```python
from build123d import *

# Parameters (mm, degrees)
F0_W     = 63.5
F0_H     = 139.7
F1_DEPTH = 5.207
F2_W     = 5.207
F2_H     = 16.9333164
F2_H_2   = 12.7
F2_H_3   = 19.05
F2_W_2   = 15.875
F2_H_4   = 5.207
F2_W_3   = 12.7
F2_W_4   = 9.525
F3_DEPTH = 5.208


# Not quite as in the source:
# - a feature names something its author has since deleted; it is built from what else it names


with BuildPart() as f1:
    # F0 (on Right) → F1 (new body)
    with BuildSketch(Plane.YZ):
        Rectangle(F0_W, F0_H)
    extrude(amount=F1_DEPTH)

    # F2 (on face) → F3 (cut, through all)
    with BuildSketch(Plane.YZ.offset(5.207)):
        with Locations((-29.1465, 41.3046418)):
            Rectangle(F2_W, F2_H)
        with Locations((-29.1465, 13.7879836)):
            Rectangle(F2_W, F2_H_2)
        with Locations((-29.1465, -11.6120164)):
            Rectangle(F2_W, F2_H_2)
        with Locations((-29.1465, -40.1870164)):
            Rectangle(F2_W, F2_H_3)
        with Locations((-23.8125, -67.2465)):
            Rectangle(F2_W_2, F2_H_4)
        with Locations((3.175, -67.2465)):
            Rectangle(F2_W_3, F2_H_4)
        with Locations((26.9875, -67.2465)):
            Rectangle(F2_W_4, F2_H_4)
        with Locations((26.9875, 67.2465)):
            Rectangle(F2_W_4, F2_H_4)
        with Locations((3.175, 67.2465)):
            Rectangle(F2_W_3, F2_H_4)
        with Locations((-23.8125, 67.2465)):
            Rectangle(F2_W_2, F2_H_4)
    extrude(amount=-F3_DEPTH, mode=Mode.SUBTRACT)


solid = f1.part
```
Could you check a few things on this model? Use its own coordinates, in mm. A direction names the side the tool comes from. Round coordinates to 2 decimals unless told otherwise and drop trailing zeros. Write each loop counter-clockwise with the first axis right and the second up, starting at its lowest first coordinate (ties: lowest second). Pieces come first, ordered by that corner, then holes. Notation, with made-up numbers: M 39.5,69 L 87.5,69 A27 cw 87.5,100 Z; hole C 16,-40 d4. An arc over 180 degrees is marked long. Write each question's results on one line, items separated by ' | '. Start each with the question number.
1. On a 3-axis mill with a long thin cutter (end or side, diameter ignored), from which of +Z, -Z, +X, -X, +Y, -Y can I reach the whole of each face in a straight line? I mean faces 1 (the face through (3, 22.225, 67)), 2 (the face through (3, -24, 64.643)), 3 (the face through (3, 22.225, -67)), 4 (the face through (3, -29, -17.962)). Say none if no direction works.
2. I need wall thicknesses on L1, parallel to Y at x = 4.95, z = 34; L2, parallel to Z at x = 4.95, y = -22. Which ranges of each line are inside material? Lowest first, please. Write a range as from..to.
3. Imagine slicing it at B-B on y = -21. List the corners of the cut face in (x, z) for me, and give its area (3 significant figures).
4. I'm going to push flat-ended pins straight in: pin 1 Ø1.6 at (x, z) = (2.5, -40) entering from -Y; pin 2 Ø2.5 at (x, y) = (3.5, 26) entering from -Z; pin 3 Ø1.6 at (x, z) = (2, -68) entering from -Y (3 decimals). Where does each tip first touch, or does it pass through?
5. Thinking about a two-plate mould opening in Y: for faces 5 (the face through (3, -29, 20.138)), 6 (the face through (3, -31.75, -24)), 7 (the face through (3, -3.175, -67)), 8 (the face through (3, 3, 64.643)), which applies, +Y half, -Y half, draft (parallel to the pull), parting line (faces both ways), or undercut?
6. Imagine slicing it at A-A on z = 40. List the corners of the cut face in (x, y) for me.
Result sheet:
1) face 1: +Z, +X, -X, +Y | face 2: +Z, +X, -X, -Y | face 3: -Z, +X, -X, +Y | face 4: +X, -X, -Y
2) L1: y = -26.54..31.75 | L2: z = -64.64..64.64
3) outline: M 0,-64.64 L 5.21,-64.64 L 5.21,64.64 L 0,64.64 Z | area: 673 mm^2
4) pin 1: stops at y = -26.54 | pin 2: stops at z = -64.64 | pin 3: stops at y = -15.875
5) face 5: draft | face 6: -Y half | face 7: undercut | face 8: undercut
6) outline: M 0,-26.54 L 5.21,-26.54 L 5.21,31.75 L 0,31.75 Z
